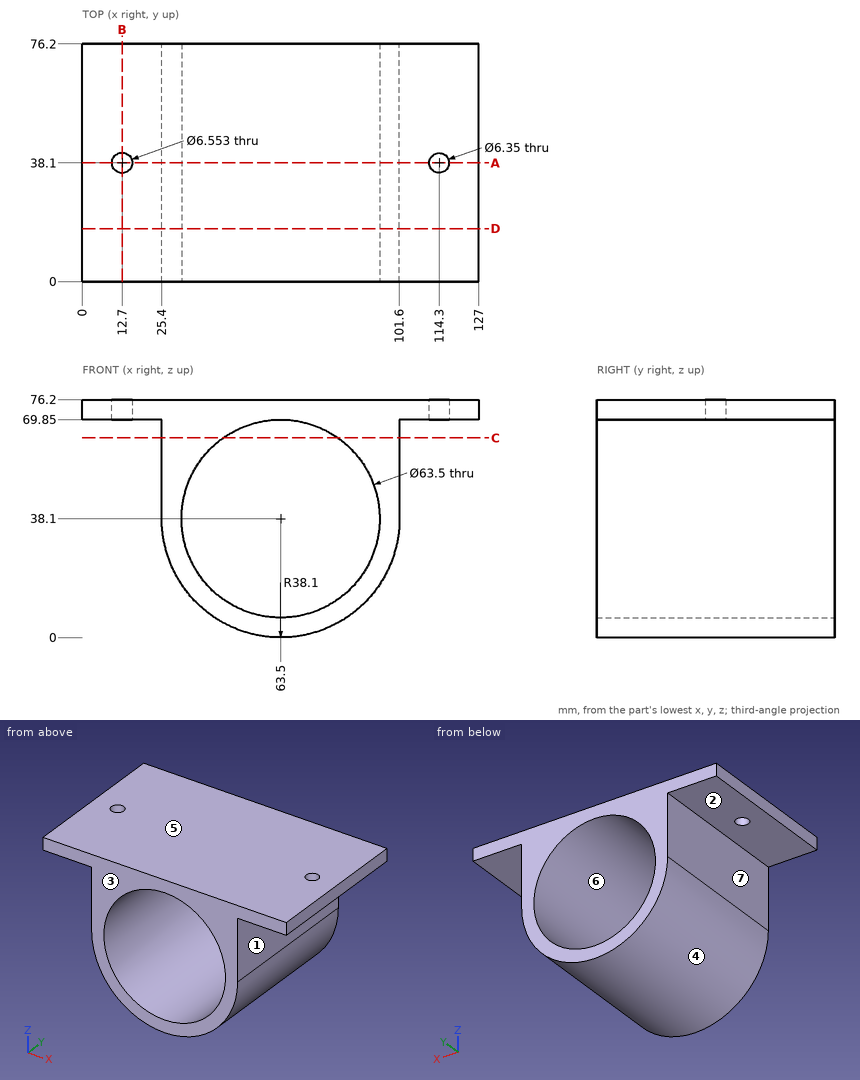
Drawing for the job (mm, zero at the part's lowest x, y, z). A direction names the side the tool comes from. Round coordinates to 2 decimals unless told otherwise and drop trailing zeros. Loops run counter-clockwise (first coordinate to the right, second up) from the corner with the lowest first, then second, coordinate; pieces in that order, holes last. Notation, with made-up numbers: (17.5, 34.5) -> (51.5, 34.5) arc R16 ccw to (51.5, 61.5) -> close; hole circle Ø6 at (-3, 48). An arc over 180 degrees is marked (long way). Use one line per item in the form item = value. Start each with the question number.
Item 1: Band-saw the part on C-C (z = 64). List the corners of the cut face in (x, y).
Item 2: Drill centre lines: line 1 along X through (y, z) = (58, 38); line 2 along Y through (x, z) = (114.3, 72.75) (3 decimals); line 3 along Z through (x, y) = (78, 12) (1 decimal). Where is each one in solid material? Low to high.
Item 3: Drop flat-ended pins along their axis: pin 1 Ø5.5 at (x, y) = (114.3, 38.1) entering from -Z (3 decimals); pin 2 Ø2 at (y, z) = (68, 57) entering from +X; pin 3 Ø12 at (x, y) = (72.5, 28.5) entering from -Z; pin 4 Ø1 at (y, z) = (65.5, 64.5) entering from -X. Give the stop position or say it passes through.
Item 4: Two-plate mould, pull along Z, no slides. Class the marked faces 4, 5, 6 and 7: released by +Z, released by -Z, zero draft, split by the parting line, or undercut.
Item 5: Band-saw the part on A-A (y = 38.1). Give the number of separate pieces and of enclosed holes in the cut face, plus the area to 3 significant figures.
Item 6: Tool access for the marked faces 1, 2 and 3: list every direction of +Z, -Z, +X, -X, +Y, -Y with a clear straight run to the whole face (end or side of a thin tool).
Item 7: Band-saw the part on D-D (y = 17). List the corners of the cut face in (x, z), plus the area to 3 significant figures.
Item 8: Band-saw the part on B-B (x = 12.7). List the corners of the cut face in (y, z), plus the area to 3 significant figures.
Data:
q1.outline = (25.4, 0) -> (45.14, 0) -> (45.14, 76.2) -> (25.4, 76.2) -> close; (81.86, 0) -> (101.6, 0) -> (101.6, 76.2) -> (81.86, 76.2) -> close
q2.line_1 = 25.4 to 31.75, 95.25 to 101.6
q2.line_2 = 0 to 34.925, 41.275 to 76.2
q2.line_3 = 2.9 to 9.9, 66.3 to 76.2
q3.pin_1 = through
q3.pin_2 = 101.6
q3.pin_3 = 0.12
q3.pin_4 = 25.4
q4.face_4 = released by -Z
q4.face_5 = released by +Z
q4.face_6 = undercut
q4.face_7 = zero draft
q5.separate_pieces = 3
q5.enclosed_holes = 1
q5.area = 2,260 mm^2
q6.face_1 = -Z, +X, +Y, -Y
q6.face_2 = -Z, -X, +Y, -Y
q6.face_3 = +Z, -Z, +X, -X, -Y
q7.outline = (0, 69.85) -> (25.4, 69.85) -> (25.4, 38.1) arc R38.1 ccw to (101.6, 38.1) -> (101.6, 69.85) -> (127, 69.85) -> (127, 76.2) -> (0, 76.2) -> close; hole circle Ø63.5 at (63.5, 38.1)
q7.area = 2,340 mm^2
q8.outline = (0, 69.85) -> (34.82, 69.85) -> (34.82, 76.2) -> (0, 76.2) -> close; (41.38, 69.85) -> (76.2, 69.85) -> (76.2, 76.2) -> (41.38, 76.2) -> close
q8.area = 442 mm^2
